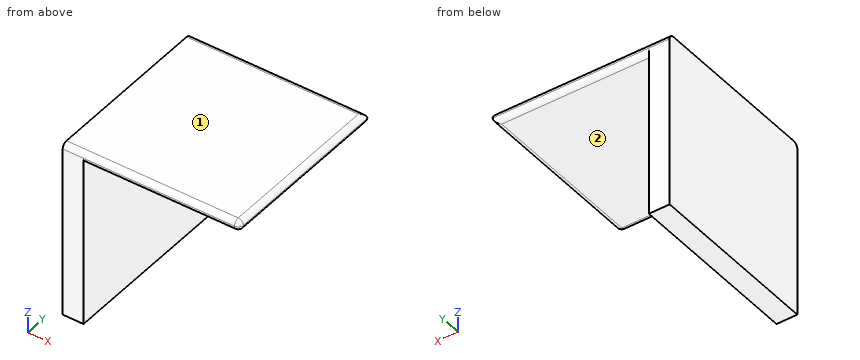
```python
from build123d import *

# Parameters (mm, degrees)
F0_W     = 431.8
F0_H     = 25.4
F1_DEPTH = 431.8
F0_H_2   = 406.4
F2_DEPTH = 50.8
F3_R     = 12.69999


# Not quite as in the source:
# - a fillet or chamfer is up to 0.001 mm smaller than in the source, because OpenCascade refuses the exact size


with BuildPart() as f1:
    # F0 (on Right) → F1 (new body)
    with BuildSketch(Plane.YZ):
        with Locations((0, 203.2)):
            Rectangle(F0_W, F0_H)
    extrude(amount=F1_DEPTH)

    # F0 (on Right) → F2 (join)
    with BuildSketch(Plane.YZ):
        with Locations((0, -12.7)):
            Rectangle(F0_W, F0_H_2)
    extrude(amount=F2_DEPTH)

    # F3 (radius 12.7 in the source; OpenCascade refuses exactly that, so slightly less here)
    f3_edges = [f1.edges().sort_by_distance(p)[0] for p in [
        (431.8, 0, 190.5),
        (431.8, -215.9, 203.2),
        (241.3, -215.9, 190.5),
        (215.9, -215.9, 215.9),
        (431.8, 0, 215.9),
        (215.9, 215.9, 215.9),
        (241.3, 215.9, 190.5),
    ]]
    fillet(f3_edges, radius=F3_R)


solid = f1.part
```
Source: CAD feature listing. Evaluate the final solid. Frame: model axes, mm. Face numbers are marked on the shaded views. A direction names the side the tool comes from. Coordinates: 2 decimals unless noted, no trailing zeros. Loops run counter-clockwise (first coordinate to the right, second up) from the corner with the lowest first, then second, coordinate; pieces in that order, holes last. Notation, with made-up numbers: (14.5, 44) -> (47.5, 44) arc R15 ccw to (47.5, 56) -> close; hole circle Ø3 at (64.5, 20.25). An arc over 180 degrees is marked (long way). One line per item, written item: value. Start each with the question number.
Q1. Set-up query: the marked faces 1 and 2. Return all of +Z, -Z, +X, -X, +Y, -Y with unobstructed straight access to the full face (end or side cutting, diameter ignored); none if empty.
Q2. Line query: line 1 along X through (y, z) = (98, 178); line 2 along Z through (x, y) = (409, -170); line 3 along X through (y, z) = (-124.5, 192). Output: solid intervals per line, ascending.
Q3. Section query C-C, the plane z = -179. Return the cut outline in (x, y), and give its area (3 significant figures).
Q4. Contact query for flat-ended pins moving along their axis: P1, Ø3, axis at x = 137, y = -46, coming from the -Z side; P2, Ø12, axis at y = -168.5, z = 72, coming from the +X side; P3, Ø12, axis at y = 129.5, z = -54, coming from the -X side. Output: stop coordinate, or through.
Results:
1. face 1: +Z, +X, -X, +Y, -Y
1. face 2: -Z, +X, +Y, -Y
2. line 1: 0 to 50.8
2. line 2: 190.5 to 215.9
2. line 3: 0 to 425.09
3. outline: (0, -215.9) -> (50.8, -215.9) -> (50.8, 215.9) -> (0, 215.9) -> close
3. area: 21,900 mm^2
4. P1: z = 190.5
4. P2: x = 50.8
4. P3: x = 0
